Input: part model. Units: mm. Frame: model coordinates. Round coordinates to 2 decimals unless told otherwise and drop trailing zeros. Order: outer loops, then holes, each group sorted by start corner. A loop starts at its lowest first (then second) coordinate and runs counter-clockwise, first axis right, second up. Notation, with made-up numbers: (19, -21.5) -> (59, -21.5) arc R28 ccw to (59, 10.5) -> close; hole circle Ø1 at (82, 37). An arc over 180 degrees is marked (long way). Answer as CSV lines item,"result". Start each with the question number.
1) Section query C-C, the plane x = 50. Output: boundary loops of the cut face in (y, z).
2) Section query D-D, the plane y = -14. Output: boundary loops of the cut face in (x, z), and give its area (3 significant figures).
3) Section query B-B, the plane y = 35.5. Output: boundary loops of the cut face in (x, z), and give its area (3 significant figures).
4) Line query: L1, parallel to Y at x = 0, z = 4; L2, parallel to X at y = 34, z = 4.4; L3, parallel to X at y = -12, z = 3.55. Output: solid intervals per line, ascending.
5) Mould query, pull axis Y, two halves, no side actions, for faces 1 (the face through (31, 9.76, 2.46)), 2 (the face through (-1, -67.5, 2)), 3 (the face through (-31, 16, 0)). Classes: +Y half, -Y half, draft (parallel to the pull), parting line (faces both ways), or undercut.
6) Section query A-A, the plane x = 0. Output: boundary loops of the cut face in (y, z), and give its area (3 significant figures).
```python
from build123d import *

# Parameters (mm, degrees)
ESBO_O1_W                = 135
ESBO_O1_H                = 135
ESBO_O1_R                = 5.178334598
ESBO_O1_R_2              = 32.5
ESBO_O1_R_3              = 4.576992867
RESSALTO_EXTRUS_O3_DEPTH = 5


with BuildPart() as part:
    # Esboço1 → Ressalto-extrusão3 (new body)
    with BuildSketch(Plane.XY):
        Rectangle(ESBO_O1_W, ESBO_O1_H)
        with Locations((-57.5, 57.5)):
            Circle(ESBO_O1_R, mode=Mode.SUBTRACT)
        with Locations(Location((-57.5, -57.5, 0), (0, 0, 180))):
            Circle(ESBO_O1_R, mode=Mode.SUBTRACT)
        with Locations((57.5, -57.5)):
            Circle(ESBO_O1_R, mode=Mode.SUBTRACT)
        with Locations(Location((57.5, 57.5, 0), (0, 0, 180))):
            Circle(ESBO_O1_R, mode=Mode.SUBTRACT)
        Circle(ESBO_O1_R_2, mode=Mode.SUBTRACT)
        with Locations((0, 52.5)):
            Circle(ESBO_O1_R_3, mode=Mode.SUBTRACT)
        with Locations((41.04615283, 32.733214598)):
            Circle(ESBO_O1_R_3, mode=Mode.SUBTRACT)
        with Locations((51.18371539, -11.682349033)):
            Circle(ESBO_O1_R_3, mode=Mode.SUBTRACT)
        with Locations((22.778896304, -47.300865565)):
            Circle(ESBO_O1_R_3, mode=Mode.SUBTRACT)
        with Locations((-22.778896304, -47.300865565)):
            Circle(ESBO_O1_R_3, mode=Mode.SUBTRACT)
        with Locations((-51.18371539, -11.682349033)):
            Circle(ESBO_O1_R_3, mode=Mode.SUBTRACT)
        with Locations((-41.04615283, 32.733214598)):
            Circle(ESBO_O1_R_3, mode=Mode.SUBTRACT)
    extrude(amount=RESSALTO_EXTRUS_O3_DEPTH)


solid = part.part
```
Findings:
1,outline,"(-67.5, 0) -> (-16.1, 0) -> (-16.1, 5) -> (-67.5, 5) -> close; (-7.26, 0) -> (67.5, 0) -> (67.5, 5) -> (-7.26, 5) -> close"
2,outline,"(-67.5, 0) -> (-55.13, 0) -> (-55.13, 5) -> (-67.5, 5) -> close; (-47.24, 0) -> (-29.33, 0) -> (-29.33, 5) -> (-47.24, 5) -> close; (29.33, 0) -> (47.24, 0) -> (47.24, 5) -> (29.33, 5) -> close; (55.13, 0) -> (67.5, 0) -> (67.5, 5) -> (55.13, 5) -> close"
2,area,"303 mm^2"
3,outline,"(-67.5, 0) -> (-44.69, 0) -> (-44.69, 5) -> (-67.5, 5) -> close; (-37.4, 0) -> (37.4, 0) -> (37.4, 5) -> (-37.4, 5) -> close; (44.69, 0) -> (67.5, 0) -> (67.5, 5) -> (44.69, 5) -> close"
3,area,"602 mm^2"
4,L1,"y = -67.5 to -32.5, 32.5 to 47.92, 57.08 to 67.5"
4,L2,"x = -67.5 to -45.44, -36.65 to 36.65, 45.44 to 67.5"
4,L3,"x = -67.5 to -55.75, -46.62 to -30.2, 30.2 to 46.62, 55.75 to 67.5"
5,face 1,"undercut"
5,face 2,"-Y half"
5,face 3,"draft"
6,outline,"(-67.5, 0) -> (-32.5, 0) -> (-32.5, 5) -> (-67.5, 5) -> close; (32.5, 0) -> (47.92, 0) -> (47.92, 5) -> (32.5, 5) -> close; (57.08, 0) -> (67.5, 0) -> (67.5, 5) -> (57.08, 5) -> close"
6,area,"304 mm^2"
